For this review, take the finished solid that the model builds, in its own axes (mm). A direction names the side the tool comes from. Round coordinates to 2 decimals unless told otherwise and drop trailing zeros. Loops run counter-clockwise (first coordinate to the right, second up) from the corner with the lowest first, then second, coordinate; pieces in that order, holes last.
```python
from build123d import *

# Parameters (mm, degrees)
EXTRUDE_THIN1_DEPTH = 12.5


with BuildPart() as part:
    # Sketch1 → Extrude-Thin1 (new, symmetric)
    with BuildSketch(Plane.XY):
        with BuildLine():
            Line((-63.809554967, 0), (0, 0))
            ThreePointArc((0, 0), (5.904048089, 7.068745133), (-2.103307553, 11.61926128))
            Line((-2.103307553, 11.61926128), (-31.409124045, 0.65))
            Line((-31.409124045, 0.65), (-61.409124045, 0.65))
            Line((-61.409124045, 0.65), (-61.409124045, 2.65))
            Line((-61.409124045, 2.65), (-31.77116213, 2.65))
            Line((-31.77116213, 2.65), (-2.804410071, 13.492348374))
            ThreePointArc((-2.804410071, 13.492348374), (7.872064119, 7.424993511), (0, -2))
            Line((0, -2), (-63.809554967, -2))
            Line((-63.809554967, -2), (-63.809554967, 0))
        make_face()
    extrude(amount=EXTRUDE_THIN1_DEPTH, both=True)


solid = part.part
```
(1) Add section B-B (y = 6). Give the boundary of the cut face in (x, z), plus the area to 3 significant figures.
(2) Insertion check: pin 1 Ø8 at (x, z) = (-41.5, -9.5) entering from +Y; pin 2 Ø8 at (y, z) = (1, -5) entering from +X; pin 3 Ø0.6 at (y, z) = (2, -5.5) entering from -X; pin 4 Ø6 at (x, y) = (0, 5.5) entering from -Z. Each pin has a flat end and moves straight along its axis. Give the tip position at first contact, or say it passes through.
(3) For faces 1 (the flat face through (-47, 2.65, 0)), 2 (the flat face through (-32, 0, 0)), 3 (the cylindrical face through (5.93, 6.92, 0.18)), list the 3-axis set-ups (+Z, -Z, +X, -X, +Y, -Y) from which the entire face can be reached by the end or side of a thin tool; tool diameter is ignored.
(4) Add section C-C (z = 0.25). Give the boundary of the cut face in (x, y), plus the area to 3 significant figures.
(5) Add section A-A (x = -49.5). Give the boundary of the cut face in (y, z).
(6) For L1, parallel to Y at x = -44.5, z = 4; L2, parallel to Y at x = -13, z = 8.25, list the stretches that pass through material, from the lowest coordinate up.
(7) The part is to be moulded in two halves that separate along X. For faces 4 (the flat face through (-16.55, 6.21, 0.18)), 5 (the flat face through (-63.81, -1, 0)), 6 (the flat face through (-25, 4, -12.5)), say which applies: pulls with the +X half, pulls with the -X half, needs draft (parallel to the pull), parting line crosses it, or undercut.
Outcome:
1. outline: (-22.82, -12.5) - (-17.12, -12.5) - (-17.12, 12.5) - (-22.82, 12.5) - close; (6, -12.5) - (8, -12.5) - (8, 12.5) - (6, 12.5) - close
1. area: 193 mm2
2. pin 1: stops at y = 2.65
2. pin 2: stops at x = 7.94
2. pin 3: stops at x = -61.41
2. pin 4: passes through
3. face 1: +Z, -Z, -X, +Y
3. face 2: +Z, -Z, -X
3. face 3: +Z, -Z
4. outline: (-63.81, -2) - (0, -2) arc R8 ccw (long way) to (-2.8, 13.49) - (-31.77, 2.65) - (-61.41, 2.65) - (-61.41, 0.65) - (-31.41, 0.65) - (-2.1, 11.62) arc R6 cw (long way) to (0, 0) - (-63.81, 0) - close
4. area: 298 mm2
5. outline: (-2, -12.5) - (0, -12.5) - (0, 12.5) - (-2, 12.5) - close; (0.65, -12.5) - (2.65, -12.5) - (2.65, 12.5) - (0.65, 12.5) - close
6. L1: y = -2 to 0, 0.65 to 2.65
6. L2: y = -2 to 0, 7.54 to 9.68
7. face 4: undercut
7. face 5: pulls with the -X half
7. face 6: needs draft
